Study the drawing (mm; zero at the part's minimum x, y, z) and answer. A direction names the side the tool comes from. Coordinates: 2 decimals unless noted, no trailing zeros. Write each loop counter-clockwise with the first axis right and the second up, starting at its lowest first coordinate (ties: lowest second). Pieces come first, ordered by that corner, then holes. Notation, with made-up numbers: (32, 49.5) -> (36, 49.5) arc R28 ccw to (36, 83.5) -> close; hole circle Ø11 at (28, 34.5). An arc over 180 degrees is marked (long way). Write item = value, one per line. Start each with the question number.
1) Section B-B (y = 6.35) is taken. Determine the outline of the cut face in (x, z) (3 decimals).
2) Section C-C (z = 20) is taken. Determine the outline of the cut face in (x, y).
3) Section D-D (z = 2.5) is taken. Determine the outline of the cut face in (x, y) (3 decimals).
4) Find the intervals of material crossed by line 1 along Y through (x, z) = (6.35, 27.5); line 2 along Y through (x, z) = (6.35, 7.5) (3 decimals); line 3 along X through (y, z) = (7.75, 10.5), in increasing order. Write a range as from..to.
5) Section A-A (x = 6.35) is taken. Determine the outline of the cut face in (y, z) (3 decimals).
6) A tool of negligible diameter and unlimited length cuts with its end or side. For the marked faces 1, 2 and 3, from which of +Z, -Z, +X, -X, +Y, -Y can it reach the whole face along a straight path? Write none if from no direction.
7) Flat-ended cylindrical pins translate along their axes: pin 1 Ø1.9 at (x, y) = (5, 5.5) entering from -Z; pin 2 Ø1 at (y, z) = (7, 23.5) entering from +X; pin 3 Ø4 at (x, z) = (2.5, 6) entering from -Y; pin 4 Ø5 at (x, z) = (2.5, 21.5) entering from +Y. Find the tip coordinate at first contact, or state that the pin passes through.
8) For a pull along X with two mould halves and no side action, classify the marked faces 4, 5 and 6 as released by +X, released by -X, zero draft, split by the parting line, or undercut.
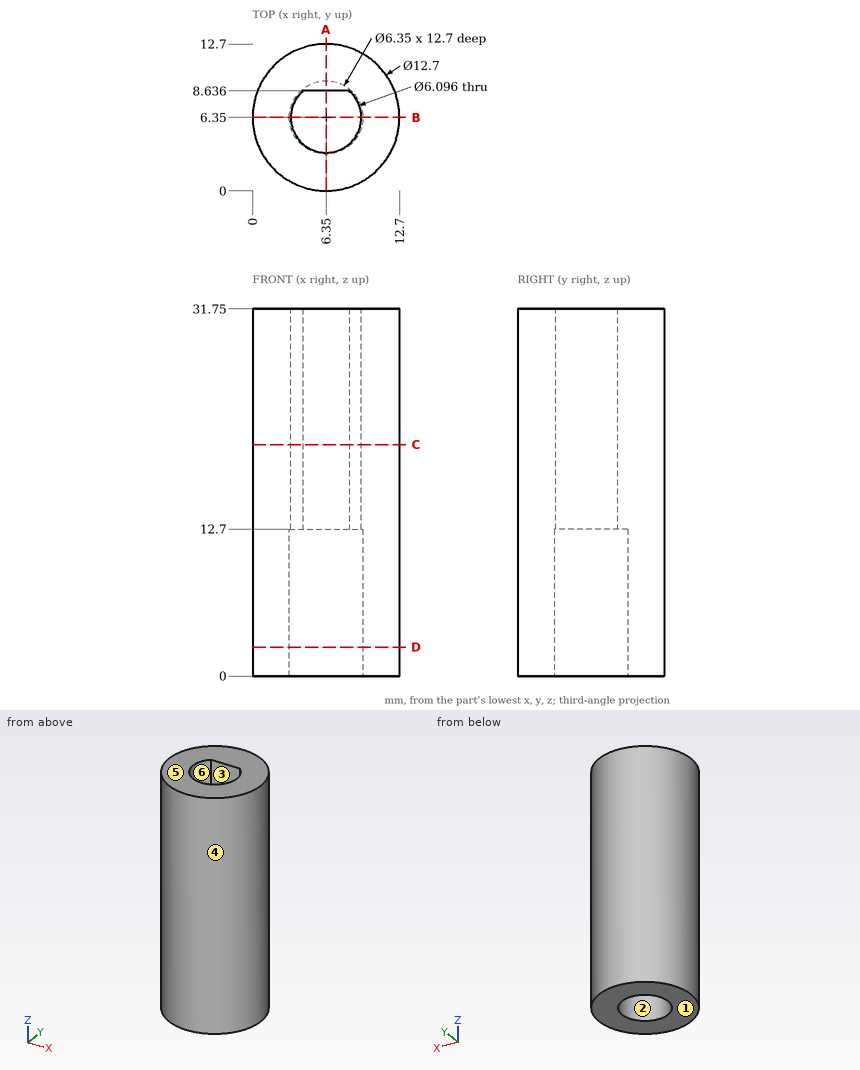
Answer key:
q1.outline = (0, 0) -> (3.175, 0) -> (3.175, 12.7) -> (3.302, 12.7) -> (3.302, 31.75) -> (0, 31.75) -> close; (9.398, 12.7) -> (9.525, 12.7) -> (9.525, 0) -> (12.7, 0) -> (12.7, 31.75) -> (9.398, 31.75) -> close
q2.outline = circle Ø12.7 at (6.35, 6.35); hole (4.33, 8.64) arc R3.05 ccw (long way) to (8.37, 8.64) -> close
q3.outline = circle Ø12.7 at (6.35, 6.35); hole circle Ø6.35 at (6.35, 6.35)
q4.line_1 = 0..3.3, 8.64..12.7
q4.line_2 = 0..3.175, 9.525..12.7
q4.line_3 = 0.16..3.5, 9.2..12.54
q5.outline = (0, 0) -> (3.175, 0) -> (3.175, 12.7) -> (3.302, 12.7) -> (3.302, 31.75) -> (0, 31.75) -> close; (8.636, 12.7) -> (9.525, 12.7) -> (9.525, 0) -> (12.7, 0) -> (12.7, 31.75) -> (8.636, 31.75) -> close
q6.face_1 = -Z, +X, -X, +Y, -Y
q6.face_2 = -Z
q6.face_3 = +Z, -Z
q7.pin_1 = through
q7.pin_2 = 12.7
q7.pin_3 = 0.28
q7.pin_4 = 12.55
q8.face_4 = split by the parting line
q8.face_5 = zero draft
q8.face_6 = undercut
